Autodesk Inventor part; units mm, degrees
ref_plane "YZ Plane" through (0, 0, 0) normal (1, 0, 0) x (0, 1, 0)
ref_plane "XZ Plane" through (0, 0, 0) normal (0, 1, 0) x (-1, 0, 0)
ref_plane "XY Plane" through (0, 0, 0) normal (0, 0, 1) x (1, 0, 0)
sketch "Sketch1" plane through (0, 0, 0) normal (0, 1, 0) x (-1, 0, 0)
  line L0 (0, 0) -> (0, -160) construction
  line L1 (5, 0) -> (5, -160)
  line L2 (-5, -160) -> (-5, 0)
  arc A0 (5, 0) -> (-5, 0) centre (0, 0) ccw
  arc A1 (-5, -160) -> (5, -160) centre (0, -160) ccw
  circle A2 centre (0, 0) radius 1.65
  line L3 (0, -30) -> (0, -120) construction
  line L4 (1.65, -30) -> (1.65, -120)
  line L5 (-1.65, -120) -> (-1.65, -30)
  arc A3 (1.65, -30) -> (-1.65, -30) centre (0, -30) ccw
  arc A4 (-1.65, -120) -> (1.65, -120) centre (0, -120) ccw
  point P0 (0, -80)
  point P1 (0, -75)
  dimension "d0" = 160
  dimension "d1" = 10
  dimension "d2" = 3.3
  dimension "d3" = 30
  dimension "d5" = 120
  dimension "d6" = 3.3
extrude "Extrusion1" add sketch "Sketch1" along normal blind 6
sketch "Sketch2" plane through (5, 0, 0) normal (1, 0, 0) x (0, 0, -1)
  line L0 (160, 0) -> (160, 6)
  line L1 (0, 0) -> (160, 0)
  line L2 (160, 0) -> (160, 6)
  line L3 (0, 6) -> (160, 6)
  line L4 (0, 0) -> (0, 6)
  line L5 (160, 0) -> (160, 0)
  line L6 (160, 0) -> (160, 6)
  line L7 (160, 6) -> (160, 6)
  line L8 (160, 0) -> (160, 6)
  line L9 (160, 0) -> (0, 0)
  arc A0 (373.775, -84) -> (160, 0) centre (160, -314.0223) ccw
  line L10 (160, 6) -> (0, 6)
  arc A1 (373.775, -78) -> (160, 6) centre (160, -308.0223) ccw
  line L11 (373.775, -78) -> (373.775, -84)
  line L12 (0, 0) -> (160, 0)
  dimension "d9" = 6
  dimension "d10" = 373.775
  dimension "d11" = 90
extrude "Extrusion2" add sketch "Sketch2" against normal blind 10 contours L0 A1 L11 A0
fillet "Fillet1" radius 2 4 edges at (0, -78, -373.775) (5, -81, -373.775) (-5, -81, -373.775) (0, -84, -373.775)
sketch "Sketch3" plane through (0, 6, 0) normal (0, 1, 0) x (1, 0, 0)
  line L0 (36.6774, -16.9321) -> (-64.8889, -16.9321)
  line L1 (-64.8889, -16.9321) -> (-64.8889, 211.3912)
  line L2 (-64.8889, 211.3912) -> (36.6774, 211.3912)
  line L3 (36.6774, 211.3912) -> (36.6774, -16.9321)
  line L4 (-92.1247, 397.3107) -> (101.238, 397.3107)
  line L5 (101.238, 397.3107) -> (101.238, -55.9315)
  line L6 (101.238, -55.9315) -> (-92.1247, -55.9315)
  line L7 (-92.1247, -55.9315) -> (-92.1247, 397.3107)
  point P0 (0, 0)
extrude "Extrusion3" cut sketch "Sketch3" against normal blind 100
properties part number "Part_11_p2"
Model file for the job. Use its own axes, mm. A direction names the side the tool comes from. Give positions to 0.01 mm unless a question says otherwise; leave off trailing zeros. Order: outer loops, then holes, each group sorted by start corner. A loop starts at its lowest first (then second) coordinate and runs counter-clockwise, first axis right, second up.
1) Saw through at C-C, the plane z = -184. Write the cut outline in (x, y).
2) Saw through at B-B, the plane z = -85.5. Write the cut outline in (x, y), then the cut area to 3 significant figures.
3) Pin check, flat tip, straight feed: pin 1 (5 mm diameter, centred on x = 1.5, z = -72.5, fed in from -Y). Stop position of the tip, or through.
4) 3-axis set-ups, long thin cutter, end or side, ignore diameter. For faces 1 (the flat face through (5, 3, -107)), 2 (the flat face through (-1.65, 3, -74)): which of +Z, -Z, +X, -X, +Y, -Y reach the whole face in a straight line?
5) Saw through at A-A, the plane x = 0. Count the separate pieces of the cut face and the enclosed holes in it, then the cut area to 3 significant figures.
6) Wall check: probe 1 along Z at (x, y) = (-0.25, 0.25); probe 2 along X at (y, z) = (0.75, -102); probe 3 along Y at (x, z) = (-2, -5). Give the ranges that are in metal, low to high.
7) Mould opens along Z. For faces 3 (the cylindrical face through (0.07, 4.91, -186.14)), 4 (the cylindrical face through (-0.04, 2.96, -121.65)), 5 (the flat face through (-2, 0, -76)) say: +Z half, -Z half, draft (parallel to the pull), parting line (faces both ways), or undercut.
Computed:
1. outline: (-5, -0.92) - (5, -0.92) - (5, 5.08) - (-5, 5.08) - close
2. outline: (-5, 0) - (-1.65, 0) - (-1.65, 6) - (-5, 6) - close; (1.65, 0) - (5, 0) - (5, 6) - (1.65, 6) - close
2. area: 40.2 mm2
3. pin 1: stops at y = 0
4. face 1: +Z, -Z, +X, +Y, -Y
4. face 2: +Y, -Y
5. separate pieces: 3
5. enclosed holes: 0
5. area: 719 mm2
6. probe 1: z = -211.39 to -121.63, -28.37 to -1.63, 1.63 to 4.99
6. probe 2: x = -5 to -1.65, 1.65 to 5
6. probe 3: y = 0 to 6
7. face 3: -Z half
7. face 4: undercut
7. face 5: draft
